from build123d import *


with BuildPart() as part:
    # Sketch3 → Revolve1 (revolve)
    with BuildSketch(Plane(origin=(0, 0, 0), x_dir=(0, 0, -1), z_dir=(1, 0, 0)), mode=Mode.PRIVATE) as revolve1_sk:
        with BuildLine():
            Line((-7.25, 44.75), (-7.25, 12.75))
            Line((-7.25, 12.75), (-137.25, 12.75))
            ThreePointArc((-137.25, 12.75), (-142.730077554, 10.480077554), (-145, 5))
            Line((-145, 5), (-150, 5))
            Line((-150, 5), (-150, 0))
            Line((-150, 0), (-145, 0))
            Line((-145, 0), (-145, -25))
            Line((-145, -25), (-150, -25))
            Line((-150, -25), (-150, -30))
            Line((-150, -30), (-145, -30))
            ThreePointArc((-145, -30), (-142.730077554, -35.480077554), (-137.25, -37.75))
            Line((-137.25, -37.75), (-7.25, -37.75))
            Line((-7.25, -37.75), (-7.25, -69.75))
            Line((-7.25, -69.75), (0, -69.75))
            Line((0, -69.75), (0, 44.75))
            Line((0, 44.75), (-7.25, 44.75))
        make_face()
    revolve(revolve1_sk.sketch.rotate(Axis((0, -69.75, 0), (0, 1, 0)), 180), axis=Axis((0, -69.75, 0), (0, 1, 0)))


solid = part.part
Can you work these out from the model? Positions are in its coordinate system, mm. A direction names the side the tool comes from. Round coordinates to 2 decimals unless told otherwise and drop trailing zeros. Write each loop counter-clockwise with the first axis right and the second up, starting at its lowest first coordinate (ties: lowest second). Pieces come first, ordered by that corner, then holes. Notation, with made-up numbers: M -9.75,-33 L 16.25,-33 A24 cw 16.25,-1 Z; hole C -8,0 d7. An arc over 180 degrees is marked long. Use a Markdown table: item, result.
Item 1: I want a section at A-A (z = 0). List the corners of the cut face in (x, y) for me, and give its area (3 significant figures).
Found:
| item | result |
|---|---|
| outline | M -150,-30 L -145,-30 A7.75 ccw -137.25,-37.75 L -7.25,-37.75 L -7.25,-69.75 L 7.25,-69.75 L 7.25,-37.75 L 137.25,-37.75 A7.75 ccw 145,-30 L 150,-30 L 150,-25 L 145,-25 L 145,0 L 150,0 L 150,5 L 145,5 A7.75 ccw 137.25,12.75 L 7.25,12.75 L 7.25,44.75 L -7.25,44.75 L -7.25,12.75 L -137.25,12.75 A7.75 ccw -145,5 L -150,5 L -150,0 L -145,0 L -145,-25 L -150,-25 Z |
| area | 15,600 mm2 |
Item 2: Which directions (+Z, -Z, +X, -X, +Y, -Y) give clear straight access to the entire face, cutting with the end or side of a thin tool? Please do faces 1 (the face through (-123, -25, -78)), 2 (the face through (133.076, -27.535, -69.216)), 3 (the face through (0, 44.75, 0)), 4 (the face through (-123, 5, -78)), 5 (the face through (6.43, -53.97, -3.35)).
Found:
| item | result |
|---|---|
| face 1 | none |
| face 2 | +Y, -Y |
| face 3 | +Z, -Z, +X, -X, +Y |
| face 4 | +Y |
| face 5 | -Y |
Item 3: For pin 1 Ø10 at (y, z) = (-0.5, -69.5) entering from -X; pin 2 Ø12 at (x, z) = (-74, -111) entering from -Y; pin 3 Ø3 at (y, z) = (-14.5, -101) entering from +X, each with a flat end and sliding along its axis, tell me the tip position at first contact or that it passes through.
Found:
| item | result |
|---|---|
| pin 1 | stops at x = -135.41 |
| pin 2 | stops at y = -37.75 |
| pin 3 | stops at x = 105.47 |
Item 4: If I drill on line 1 along Y through (x, z) = (-20.5, -56); line 2 along X through (y, z) = (-13, 97); line 3 along X through (y, z) = (-5, 36), over which ranges is the centre line in solid material (lowest first)? Write a range as [from, to].
Found:
| item | result |
|---|---|
| line 1 | y = [-37.75, 12.75] |
| line 2 | x = [-107.78, 107.78] |
| line 3 | x = [-140.46, 140.46] |
Item 5: We'd pull the mould along Y, two halves only. Please class faces 6 (the face through (-2, 12.75, 29)), 7 (the face through (128.64, -12.68, -66.91)), 8 (the face through (0, -69.75, 0)): released by +Y, released by -Y, zero draft, split by the parting line, or undercut.
Found:
| item | result |
|---|---|
| face 6 | released by +Y |
| face 7 | undercut |
| face 8 | released by -Y |
Item 6: I want a section at B-B (x = 0). List the corners of the cut face in (y, z) for me, and give its area (3 significant figures).
Found:
| item | result |
|---|---|
| outline | M -69.75,-7.25 L -37.75,-7.25 L -37.75,-137.25 A7.75 ccw -30,-145 L -30,-150 L -25,-150 L -25,-145 L 0,-145 L 0,-150 L 5,-150 L 5,-145 A7.75 ccw 12.75,-137.25 L 12.75,-7.25 L 44.75,-7.25 L 44.75,7.25 L 12.75,7.25 L 12.75,137.25 A7.75 ccw 5,145 L 5,150 L 0,150 L 0,145 L -25,145 L -25,150 L -30,150 L -30,145 A7.75 ccw -37.75,137.25 L -37.75,7.25 L -69.75,7.25 Z |
| area | 15,600 mm2 |
Item 7: I want a section at C-C (y = -19). List the corners of the cut face in (x, z) for me.
Found:
| item | result |
|---|---|
| outline | C 0,0 d290 |
